from build123d import *

# Parameters (mm, degrees)
EXTRUDE_1_DEPTH = 2


with BuildPart() as part:
    # Model → 凸台-拉伸1 (new body)
    with BuildSketch(Plane.XY):
        Polygon((973.664956946, 622.02348986), (973.664956946, 615.633131528), (978.664956946, 615.633131528), (978.664956946, 610.633131528), (973.664956946, 610.633131528), (973.664956946, 607.740854359), (972.164956946, 607.740854359), (972.164956946, 597.740854359), (973.664956946, 597.740854359), (973.664956946, 583.190731528), (972.164956946, 583.190731528), (972.164956946, 573.190731528), (973.664956946, 573.190731528), (973.664956946, 568.633131528), (978.664956946, 568.633131528), (978.664956946, 563.633131528), (983.664956946, 563.633131528), (983.664956946, 561.633131528), (993.664956946, 561.633131528), (993.664956946, 563.633131528), (998.664956946, 563.633131528), (998.664956946, 561.633131528), (1008.664956946, 561.633131528), (1008.664956946, 563.633131528), (1013.664956946, 563.633131528), (1013.664956946, 568.633131528), (1018.664956946, 568.633131528), (1018.664956946, 573.190731528), (1020.164956946, 573.190731528), (1020.164956946, 583.190731528), (1018.664956946, 583.190731528), (1018.664956946, 597.740854359), (1020.16592277, 597.740854359), (1020.16592277, 607.740854359), (1018.664956946, 607.740854359), (1018.664956946, 610.633131528), (1013.664956946, 610.633131528), (1013.664956946, 615.633131528), (1018.664956946, 615.633131528), (1018.664956946, 622.02348986), align=None)
        with BuildLine():
            Line((980.664956946, 605.633131528), (981.664956946, 605.633131528))
            ThreePointArc((981.664956946, 605.633131528), (983.079170509, 606.218917965), (983.664956946, 607.633131528))
            Line((983.664956946, 607.633131528), (983.664956946, 612.353131528))
            ThreePointArc((983.664956946, 612.353131528), (983.079170509, 613.76734509), (981.664956946, 614.353131528))
            ThreePointArc((981.664956946, 614.353131528), (980.957850165, 614.646024746), (980.664956946, 615.353131528))
            Line((980.664956946, 615.353131528), (980.664956946, 618.353131528))
            ThreePointArc((980.664956946, 618.353131528), (980.957850165, 619.060238309), (981.664956946, 619.353131528))
            Line((981.664956946, 619.353131528), (1010.664956946, 619.353131528))
            ThreePointArc((1010.664956946, 619.353131528), (1011.372063727, 619.060238309), (1011.664956946, 618.353131528))
            Line((1011.664956946, 618.353131528), (1011.664956946, 615.353131528))
            ThreePointArc((1011.664956946, 615.353131528), (1011.372063727, 614.646024746), (1010.664956946, 614.353131528))
            ThreePointArc((1010.664956946, 614.353131528), (1009.250743384, 613.76734509), (1008.664956946, 612.353131528))
            Line((1008.664956946, 612.353131528), (1008.664956946, 607.633131528))
            ThreePointArc((1008.664956946, 607.633131528), (1009.250743384, 606.218917965), (1010.664956946, 605.633131528))
            Line((1010.664956946, 605.633131528), (1011.664956946, 605.633131528))
            ThreePointArc((1011.664956946, 605.633131528), (1013.079170509, 605.04734509), (1013.664956946, 603.633131528))
            Line((1013.664956946, 603.633131528), (1013.664956946, 575.633131528))
            ThreePointArc((1013.664956946, 575.633131528), (1013.079170509, 574.218917965), (1011.664956946, 573.633131528))
            Line((1011.664956946, 573.633131528), (1010.664956946, 573.633131528))
            ThreePointArc((1010.664956946, 573.633131528), (1009.250743384, 573.04734509), (1008.664956946, 571.633131528))
            Line((1008.664956946, 571.633131528), (1008.664956946, 570.633131528))
            ThreePointArc((1008.664956946, 570.633131528), (1008.079170509, 569.218917965), (1006.664956946, 568.633131528))
            Line((1006.664956946, 568.633131528), (985.664956946, 568.633131528))
            ThreePointArc((985.664956946, 568.633131528), (984.250743384, 569.218917965), (983.664956946, 570.633131528))
            Line((983.664956946, 570.633131528), (983.664956946, 571.633131528))
            ThreePointArc((983.664956946, 571.633131528), (983.079170509, 573.04734509), (981.664956946, 573.633131528))
            Line((981.664956946, 573.633131528), (980.664956946, 573.633131528))
            ThreePointArc((980.664956946, 573.633131528), (979.250743384, 574.218917965), (978.664956946, 575.633131528))
            Line((978.664956946, 575.633131528), (978.664956946, 603.633131528))
            ThreePointArc((978.664956946, 603.633131528), (979.250743384, 605.04734509), (980.664956946, 605.633131528))
        make_face(mode=Mode.SUBTRACT)
    extrude(amount=EXTRUDE_1_DEPTH)


solid = part.part
Verification items for the finished model (mm, model axes). A direction names the side the tool comes from. Give positions to 0.01 mm unless a question says otherwise; leave off trailing zeros. Write each loop counter-clockwise with the first axis right and the second up, starting at its lowest first coordinate (ties: lowest second). Pieces come first, ordered by that corner, then holes.
(1) Mould release check, pull along X, two halves, no side actions. Record for faces 1 (the face through (976, 568.633, 1)), 2 (the face through (1009.24, 606.23, 0.99)), 3 (the face through (978.665, 566, 1)): +X half, -X half, draft (parallel to the pull), parting line (faces both ways), or undercut.
(2) Material ranges on line 1 (Y direction, x = 997.5, z = 1.55); line 2 (Y direction, x = 1005, z = 0.5); line 3 (Y direction, x = 1009.5, z = 0.85), recorded low to high.
(3) Cross-section at A-A (y = 577.5). Enter the section's corners in (x, z).
(4) Access from +Z, -Z, +X, -X, +Y, -Y to the whole of each face (thin tool, end or side, straight path). Record for faces 4 (the face through (996, 619.353, 1)), 5 (the face through (1013.665, 613, 1)), 6 (the face through (973, 583.191, 1)), 7 (the face through (1018.665, 619, 1)).
(5) Cross-section at B-B (x = 998). Enter the section's corners in (y, z), plus the area to 3 significant figures.
(6) Gauge pin test, flat ends, axial feed: pin 1 (1 mm diameter, centred on y = 609, z = 1.5, fed in from -X); pin 2 (1.2 mm diameter, centred on x = 973, z = 1, fed in from +Y); pin 3 (12 mm diameter, centred on x = 1006, y = 605.5, fed in from -Z); pin 4 (1 mm diameter, centred on y = 586, z = 1.5, fed in from +X). Record the tip position at first contact, or that the pin passes through.
Worked out:
1. face 1: draft
1. face 2: undercut
1. face 3: -X half
2. line 1: y = 563.63 to 568.63, 619.35 to 622.02
2. line 2: y = 561.63 to 568.63, 619.35 to 622.02
2. line 3: y = 563.63 to 573.26, 606.01 to 613.98, 619.35 to 622.02
3. outline: (972.16, 0) - (978.66, 0) - (978.66, 2) - (972.16, 2) - close; (1013.66, 0) - (1020.16, 0) - (1020.16, 2) - (1013.66, 2) - close
4. face 4: +Z, -Z
4. face 5: +Z, -Z, +X
4. face 6: +Z, -Z, -X
4. face 7: +Z, -Z, +X, +Y
5. outline: (563.63, 0) - (568.63, 0) - (568.63, 2) - (563.63, 2) - close; (619.35, 0) - (622.02, 0) - (622.02, 2) - (619.35, 2) - close
5. area: 15.3 mm2
6. pin 1: stops at x = 973.66
6. pin 2: stops at y = 607.74
6. pin 3: stops at z = 0
6. pin 4: stops at x = 1018.66
